Input: part model. Units: mm. Frame: model coordinates. A direction names the side the tool comes from. Round coordinates to 2 decimals unless told otherwise and drop trailing zeros. Loops run counter-clockwise (first coordinate to the right, second up) from the corner with the lowest first, then second, coordinate; pieces in that order, holes last. Notation, with made-up numbers: (-3, 56.5) - (13, 56.5) arc R26 ccw to (13, 76.5) - close; hole circle Ø7 at (2.5, 22). An arc over 180 degrees is marked (long way). One line per question, with ' | ' between items. Start each with the question number.
Item 1: Draft query along Y for faces 4 (the face through (105, 0, 3)), 5 (the face through (186.5, 259, 3)), 6 (the face through (105, 360, 3)). Return one class per face: pulls with the +Y half, pulls with the -Y half, needs draft (parallel to the pull), parting line crosses it, or undercut.
Item 2: Section A-A, the plane y = 227.5. Return loops of the section in (x, z).
Item 3: Section B-B, the plane z = 1. Return loops of the section in (x, y).
Item 4: Material intervals for line 1 along Y through (x, z) = (106.5, 1.4); line 2 along Y through (x, z) = (196.5, 1.1); line 3 along Y through (x, z) = (137, 5), sorted ascending.
Item 5: First-contact query: pin 1 (5 mm diameter, centred on x = 106, y = 352, fed in from +Z); pin 2 (1.5 mm diameter, centred on x = 52, z = 4.5, fed in from -Y); pin 3 (4 mm diameter, centred on x = 16.5, y = 240, fed in from +Z); pin 4 (2 mm diameter, centred on y = 247.5, z = 4.5, fed in from -X). Flat tips, straight axial feed; report the tip coordinate or a pass-through.
Item 6: Set-up query: faces 1 (the face through (105, 300, 3)), 2 (the face through (105, 183, 6.5)), 3 (the face through (19.3, 244.38, 4.82)). Return all of +Z, -Z, +X, -X, +Y, -Y with unobstructed straight access to the full face (end or side cutting, diameter ignored); none if empty.
```python
from build123d import *

# Parameters (mm, degrees)
SKETCH_W        = 213
SKETCH_H        = 360
PAD_DEPTH       = 6.5
SKETCH001_R     = 5.2
POCKET_DEPTH    = 3.4
SKETCH002_R     = 3.2
POCKET001_DEPTH = 3.1
FILLET_R        = 4
SKETCH003_W     = 160
SKETCH003_H     = 80
POCKET002_DEPTH = 6.5


with BuildPart() as part:
    # Sketch → Pad (new body)
    with BuildSketch(Plane.XY):
        with Locations((106.5, 180)):
            Rectangle(SKETCH_W, SKETCH_H)
    extrude(amount=PAD_DEPTH)

    # Sketch001 (on Face6 of Pad) → Pocket (cut)
    with BuildSketch(Plane.XY.offset(6.5)):
        with Locations((106.5, 350)):
            Circle(SKETCH001_R)
        with Locations((16.5, 240)):
            Circle(SKETCH001_R)
        with Locations((16.5, 120)):
            Circle(SKETCH001_R)
        with Locations((196.5, 240)):
            Circle(SKETCH001_R)
        with Locations((196.5, 120)):
            Circle(SKETCH001_R)
        with Locations((106.5, 10)):
            Circle(SKETCH001_R)
    extrude(amount=-POCKET_DEPTH, mode=Mode.SUBTRACT)

    # Sketch002 (on Face17 of Pocket) → Pocket001 (cut)
    with BuildSketch(Plane.XY.offset(3.1)):
        with Locations((106.5, 350)):
            Circle(SKETCH002_R)
        with Locations((16.5, 240)):
            Circle(SKETCH002_R)
        with Locations((16.5, 120)):
            Circle(SKETCH002_R)
        with Locations((196.5, 240)):
            Circle(SKETCH002_R)
        with Locations((196.5, 120)):
            Circle(SKETCH002_R)
        with Locations((106.5, 10)):
            Circle(SKETCH002_R)
    extrude(amount=-POCKET001_DEPTH, mode=Mode.SUBTRACT)

    # Fillet
    fillet_edges = [part.edges().sort_by_distance(p)[0] for p in [
        (213, 180, 6.5),
        (0, 180, 6.5),
    ]]
    fillet(fillet_edges, radius=FILLET_R)

    # Sketch003 (on Face5 of Fillet) → Pocket002 (cut)
    with BuildSketch(Plane.XY.offset(6.5)):
        with Locations((106.5, 260)):
            Rectangle(SKETCH003_W, SKETCH003_H)
    extrude(amount=-POCKET002_DEPTH, mode=Mode.SUBTRACT)


solid = part.part
```
Return value:
1) face 4: pulls with the -Y half | face 5: undercut | face 6: pulls with the +Y half
2) outline: (0, 0) - (26.5, 0) - (26.5, 6.5) - (4, 6.5) arc R4 ccw to (0, 2.5) - close; (186.5, 0) - (213, 0) - (213, 2.5) arc R4 ccw to (209, 6.5) - (186.5, 6.5) - close
3) outline: (0, 0) - (213, 0) - (213, 360) - (0, 360) - close; hole circle Ø6.4 at (16.5, 120); hole circle Ø6.4 at (16.5, 240); hole (26.5, 220) - (186.5, 220) - (186.5, 300) - (26.5, 300) - close; hole circle Ø6.4 at (106.5, 10); hole circle Ø6.4 at (106.5, 350); hole circle Ø6.4 at (196.5, 120); hole circle Ø6.4 at (196.5, 240)
4) line 1: 0 to 6.8, 13.2 to 220, 300 to 346.8, 353.2 to 360 | line 2: 0 to 116.8, 123.2 to 236.8, 243.2 to 360 | line 3: 0 to 220, 300 to 360
5) pin 1: z = 3.1 | pin 2: y = 0 | pin 3: through | pin 4: x = 0.13
6) face 1: +Z, -Z | face 2: +Z, +X, -X, +Y, -Y | face 3: +Z
